Verification items for the finished model (mm, model axes). Coordinates: 2 decimals unless noted, no trailing zeros. Loops run counter-clockwise (first coordinate to the right, second up) from the corner with the lowest first, then second, coordinate; pieces in that order, holes last.
Q1. Go/stop test with a flat-tipped pin: P1, Ø0.9, axis at x = 113.03, y = 77.978, coming from the -Z side. Record where the tip stops, or that it passes through.
Q2. Sectioned sample at B-B (z = -0.2). Count the separate pieces of the cut face and the enclosed holes in it, then the cut area to 3 significant figures.
Q3. Sectioned sample at A-A (y = 147). Enter the section's corners in (x, z) (3 decimals), then the cut area to 3 significant figures.
Q4. Material ranges on probe 1 along Y at (x, z) = (88.5, -0.3); probe 2 along X at (y, z) = (135, -0.25); probe 3 along Y at (x, z) = (109, -0.35), recorded low to high.
```python
from build123d import *

# Parameters (mm, degrees)
SKETCH1_R           = 0.508
SKETCH1_R_2         = 0.5999988
SKETCH1_R_3         = 0.635
SKETCH1_R_4         = 0.3999992
SKETCH1_R_5         = 0.42500042
SKETCH1_R_6         = 0.4499991
SKETCH1_R_7         = 0.4826
SKETCH1_R_8         = 1.499997
SKETCH1_R_9         = 1.4
SKETCH1_W           = 36.995943026
SKETCH1_H           = 10
BOSS_EXTRUDE1_DEPTH = 0.41148


with BuildPart() as part:
    # Sketch1 → Boss-Extrude1 (new body)
    with BuildSketch(Plane.XY):
        Polygon((70.438392982, 67.709058894), (127.180315397, 67.544049582), (127.428203039, 159.380807101), (70.428082966, 159.380807101), align=None)
        with Locations(Location((113.792, 110.998, 0), (0, 0, 180))):
            Circle(SKETCH1_R, mode=Mode.SUBTRACT)
        with Locations(Location((113.792, 113.538, 0), (0, 0, 180))):
            Circle(SKETCH1_R, mode=Mode.SUBTRACT)
        with Locations(Location((113.919, 99.8449997, 0), (0, 0, 180))):
            Circle(SKETCH1_R_2, mode=Mode.SUBTRACT)
        with Locations(Location((113.538, 103.759, 0), (0, 0, 180))):
            Circle(SKETCH1_R_3, mode=Mode.SUBTRACT)
        with Locations(Location((107.95, 99.822, 0), (0, 0, 180))):
            Circle(SKETCH1_R_4, mode=Mode.SUBTRACT)
        with Locations(Location((111.125, 98.806, 0), (0, 0, 180))):
            Circle(SKETCH1_R_5, mode=Mode.SUBTRACT)
        with Locations(Location((113.919, 89.3850003, 0), (0, 0, 180))):
            Circle(SKETCH1_R_2, mode=Mode.SUBTRACT)
        with Locations(Location((107.95, 98.552, 0), (0, 0, 180))):
            Circle(SKETCH1_R_4, mode=Mode.SUBTRACT)
        with Locations(Location((111.125, 88.646, 0), (0, 0, 180))):
            Circle(SKETCH1_R_5, mode=Mode.SUBTRACT)
        with Locations(Location((104.902, 98.806, 0), (0, 0, 180))):
            Circle(SKETCH1_R_5, mode=Mode.SUBTRACT)
        with Locations(Location((107.95, 97.282, 0), (0, 0, 180))):
            Circle(SKETCH1_R_4, mode=Mode.SUBTRACT)
        with Locations(Location((100.838, 99.695, 0), (0, 0, 180))):
            Circle(SKETCH1_R_4, mode=Mode.SUBTRACT)
        with Locations(Location((100.838, 98.425, 0), (0, 0, 180))):
            Circle(SKETCH1_R_4, mode=Mode.SUBTRACT)
        with Locations(Location((101.346, 94.234, 0), (0, 0, 180))):
            Circle(SKETCH1_R_6, mode=Mode.SUBTRACT)
        with Locations(Location((104.902, 88.646, 0), (0, 0, 180))):
            Circle(SKETCH1_R_5, mode=Mode.SUBTRACT)
        with Locations(Location((100.838, 97.155, 0), (0, 0, 180))):
            Circle(SKETCH1_R_4, mode=Mode.SUBTRACT)
        with Locations(Location((101.346, 86.614, 0), (0, 0, 180))):
            Circle(SKETCH1_R_6, mode=Mode.SUBTRACT)
        with Locations(Location((113.157, 86.106, 0), (0, 0, 180))):
            Circle(SKETCH1_R, mode=Mode.SUBTRACT)
        with Locations(Location((113.157, 83.566, 0), (0, 0, 180))):
            Circle(SKETCH1_R, mode=Mode.SUBTRACT)
        with Locations(Location((109.74201826, 82.0511948, 0), (0, 0, 180))):
            Circle(SKETCH1_R_7, mode=Mode.SUBTRACT)
        with Locations(Location((113.03, 80.518, 0), (0, 0, 180))):
            Circle(SKETCH1_R, mode=Mode.SUBTRACT)
        with Locations(Location((113.03, 74.676, 0), (0, 0, 180))):
            Circle(SKETCH1_R, mode=Mode.SUBTRACT)
        with Locations(Location((113.03, 72.136, 0), (0, 0, 180))):
            Circle(SKETCH1_R, mode=Mode.SUBTRACT)
        with Locations(Location((109.74201826, 79.5111948, 0), (0, 0, 180))):
            Circle(SKETCH1_R_7, mode=Mode.SUBTRACT)
        with Locations(Location((113.03, 77.978, 0), (0, 0, 180))):
            Circle(SKETCH1_R, mode=Mode.SUBTRACT)
        with Locations(Location((108.585, 86.487, 0), (0, 0, 180))):
            Circle(SKETCH1_R, mode=Mode.SUBTRACT)
        with Locations(Location((109.74201826, 76.9711948, 0), (0, 0, 180))):
            Circle(SKETCH1_R_7, mode=Mode.SUBTRACT)
        with Locations(Location((98.806, 86.614, 0), (0, 0, 180))):
            Circle(SKETCH1_R_6, mode=Mode.SUBTRACT)
        with Locations(Location((106.045, 86.487, 0), (0, 0, 180))):
            Circle(SKETCH1_R, mode=Mode.SUBTRACT)
        with Locations(Location((106.172, 70.866, 0), (0, 0, 180))):
            Circle(SKETCH1_R_6, mode=Mode.SUBTRACT)
        with Locations(Location((108.712, 70.866, 0), (0, 0, 180))):
            Circle(SKETCH1_R_6, mode=Mode.SUBTRACT)
        with Locations(Location((101.092, 70.866, 0), (0, 0, 180))):
            Circle(SKETCH1_R_6, mode=Mode.SUBTRACT)
        with Locations(Location((103.632, 70.866, 0), (0, 0, 180))):
            Circle(SKETCH1_R_6, mode=Mode.SUBTRACT)
        with Locations(Location((96.266, 94.234, 0), (0, 0, 180))):
            Circle(SKETCH1_R_6, mode=Mode.SUBTRACT)
        with Locations(Location((96.012, 99.949, 0), (0, 0, 180))):
            Circle(SKETCH1_R, mode=Mode.SUBTRACT)
        with Locations(Location((93.726, 94.234, 0), (0, 0, 180))):
            Circle(SKETCH1_R_6, mode=Mode.SUBTRACT)
        with Locations(Location((90.932, 99.949, 0), (0, 0, 180))):
            Circle(SKETCH1_R, mode=Mode.SUBTRACT)
        with Locations(Location((93.472, 99.949, 0), (0, 0, 180))):
            Circle(SKETCH1_R, mode=Mode.SUBTRACT)
        with Locations(Location((98.806, 94.234, 0), (0, 0, 180))):
            Circle(SKETCH1_R_6, mode=Mode.SUBTRACT)
        with Locations(Location((93.726, 86.614, 0), (0, 0, 180))):
            Circle(SKETCH1_R_6, mode=Mode.SUBTRACT)
        with Locations(Location((88.646, 94.234, 0), (0, 0, 180))):
            Circle(SKETCH1_R_6, mode=Mode.SUBTRACT)
        with Locations(Location((91.186, 94.234, 0), (0, 0, 180))):
            Circle(SKETCH1_R_6, mode=Mode.SUBTRACT)
        with Locations(Location((83.566, 104.775, 0), (0, 0, 180))):
            Circle(SKETCH1_R_3, mode=Mode.SUBTRACT)
        with Locations(Location((85.852, 99.949, 0), (0, 0, 180))):
            Circle(SKETCH1_R, mode=Mode.SUBTRACT)
        with Locations(Location((83.439, 116.332, 0), (0, 0, 180))):
            Circle(SKETCH1_R_3, mode=Mode.SUBTRACT)
        with Locations(Location((83.566, 108.966, 0), (0, 0, 180))):
            Circle(SKETCH1_R_3, mode=Mode.SUBTRACT)
        with Locations(Location((88.392, 99.949, 0), (0, 0, 180))):
            Circle(SKETCH1_R, mode=Mode.SUBTRACT)
        with Locations(Location((86.106, 94.234, 0), (0, 0, 180))):
            Circle(SKETCH1_R_6, mode=Mode.SUBTRACT)
        with Locations(Location((83.312, 99.949, 0), (0, 0, 180))):
            Circle(SKETCH1_R, mode=Mode.SUBTRACT)
        with Locations(Location((83.566, 94.234, 0), (0, 0, 180))):
            Circle(SKETCH1_R_6, mode=Mode.SUBTRACT)
        with Locations(Location((91.186, 86.614, 0), (0, 0, 180))):
            Circle(SKETCH1_R_6, mode=Mode.SUBTRACT)
        with Locations(Location((96.266, 86.614, 0), (0, 0, 180))):
            Circle(SKETCH1_R_6, mode=Mode.SUBTRACT)
        with Locations(Location((88.646, 86.614, 0), (0, 0, 180))):
            Circle(SKETCH1_R_6, mode=Mode.SUBTRACT)
        with Locations(Location((91.9620208, 79.5111948, 0), (0, 0, 180))):
            Circle(SKETCH1_R_8, mode=Mode.SUBTRACT)
        with Locations(Location((96.012, 70.866, 0), (0, 0, 180))):
            Circle(SKETCH1_R_6, mode=Mode.SUBTRACT)
        with Locations(Location((98.552, 70.866, 0), (0, 0, 180))):
            Circle(SKETCH1_R_6, mode=Mode.SUBTRACT)
        with Locations(Location((90.932, 70.866, 0), (0, 0, 180))):
            Circle(SKETCH1_R_6, mode=Mode.SUBTRACT)
        with Locations(Location((93.472, 70.866, 0), (0, 0, 180))):
            Circle(SKETCH1_R_6, mode=Mode.SUBTRACT)
        with Locations(Location((86.106, 86.614, 0), (0, 0, 180))):
            Circle(SKETCH1_R_6, mode=Mode.SUBTRACT)
        with Locations(Location((85.09, 82.042, 0), (0, 0, 180))):
            Circle(SKETCH1_R, mode=Mode.SUBTRACT)
        with Locations(Location((83.566, 86.614, 0), (0, 0, 180))):
            Circle(SKETCH1_R_6, mode=Mode.SUBTRACT)
        with Locations(Location((82.55, 82.042, 0), (0, 0, 180))):
            Circle(SKETCH1_R, mode=Mode.SUBTRACT)
        with Locations(Location((85.852, 70.866, 0), (0, 0, 180))):
            Circle(SKETCH1_R_6, mode=Mode.SUBTRACT)
        with Locations(Location((88.392, 70.866, 0), (0, 0, 180))):
            Circle(SKETCH1_R_6, mode=Mode.SUBTRACT)
        with Locations(Location((82.55, 76.708, 0), (0, 0, 180))):
            Circle(SKETCH1_R, mode=Mode.SUBTRACT)
        with Locations(Location((85.09, 76.708, 0), (0, 0, 180))):
            Circle(SKETCH1_R, mode=Mode.SUBTRACT)
        with Locations((123.36340718, 135.380807101)):
            Circle(SKETCH1_R_9, mode=Mode.SUBTRACT)
        with Locations((74.430782191, 135.380807101)):
            Circle(SKETCH1_R_9, mode=Mode.SUBTRACT)
        with Locations((74.433593858, 110.380807101)):
            Circle(SKETCH1_R_9, mode=Mode.SUBTRACT)
        with Locations((123.295926672, 110.380807101)):
            Circle(SKETCH1_R_9, mode=Mode.SUBTRACT)
        with Locations((74.436405524, 85.380807101)):
            Circle(SKETCH1_R_9, mode=Mode.SUBTRACT)
        with Locations((123.228446164, 85.380807101)):
            Circle(SKETCH1_R_9, mode=Mode.SUBTRACT)
        with Locations((98.932971513, 144.380807101)):
            Rectangle(SKETCH1_W, SKETCH1_H, mode=Mode.SUBTRACT)
    extrude(amount=-BOSS_EXTRUDE1_DEPTH)


solid = part.part
```
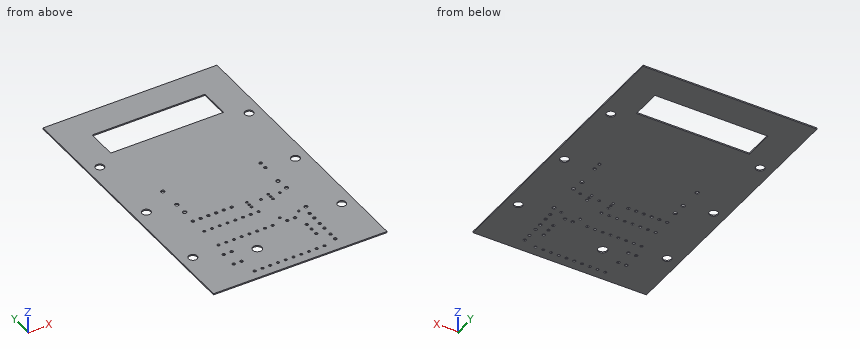
Geometry check:
1. P1: passes through
2. separate pieces: 1
2. enclosed holes: 73
2. area: 4,760 mm2
3. outline: (70.429, -0.411) - (80.435, -0.411) - (80.435, 0) - (70.429, 0) - close; (117.431, -0.411) - (127.395, -0.411) - (127.395, 0) - (117.431, 0) - close
3. area: 8.22 mm2
4. probe 1: y = 67.66 to 70.43, 71.3 to 86.19, 87.04 to 93.81, 94.66 to 99.45, 100.45 to 139.38, 149.38 to 159.38
4. probe 2: x = 70.43 to 73.08, 75.78 to 122.02, 124.71 to 127.36
4. probe 3: y = 67.6 to 70.52, 71.21 to 86.19, 86.78 to 139.38, 149.38 to 159.38
